Source: CAD feature listing. Evaluate the final solid. Frame: model axes, mm. Give positions to 0.01 mm unless a question says otherwise; leave off trailing zeros. Write each loop counter-clockwise with the first axis right and the second up, starting at its lowest first coordinate (ties: lowest second). Pieces come first, ordered by that corner, then holes. Notation, with made-up numbers: (83, -27.75) -> (110, -27.75) arc R27 ccw to (110, -11.75) -> close; hole circle Ø8 at (29.5, 15). An arc over 180 degrees is marked (long way). Answer as a JSON object with one key per item and string values. Group by question number.
Item 1: Section query B-B on x = 0. Return the cut outline in (y, z), plus the area to 3 significant figures.
Item 2: Section query A-A on y = 0. Return the cut outline in (x, z).
Item 3: First-contact query: pin 1 Ø3.5 at (x, y) = (-26.63, -8.65) entering from +Z; pin 2 Ø1.5 at (x, y) = (2, 15.5) entering from -Z; pin 3 Ø1 at (y, z) = (-8.5, 1) entering from -X; pin 4 Ø1 at (y, z) = (-23, 0.5) entering from -X. Flat tips, straight axial feed; report the tip coordinate or a pass-through.
Item 4: Pull-direction query (Y, two-part tool) for faces 1 (the face through (-2.93, -13.18, 1.97)), 2 (the face through (14, 0, 4)), 3 (the face through (31, 9.76, 1.97)); classes: pulls with the +Y half, pulls with the -Y half, needs draft (parallel to the pull), parting line crosses it, or undercut.
Item 5: Section query C-C on z = 3.1. Return the cut outline in (x, y), plus the area to 3 significant figures.
Item 6: Ray query, probe 1 along Y at (x, z) = (0, 2.2); probe 2 along X at (y, z) = (21.5, 0.8); probe 3 along X at (y, z) = (7.5, 3.15). Return the intervals inside material, ascending. Write a range as from..to.
Item 7: Section query D-D on x = 11.5. Return the cut outline in (y, z).
from build123d import *

# Parameters (mm, degrees)
SKETCH_1_R      = 32.5
SKETCH_1_R_2    = 13.5
SKETCH_1_R_3    = 2
EXTRUDE_1_DEPTH = 4


with BuildPart() as part:
    # 草图1 → 凸台-拉伸1 (new body)
    with BuildSketch(Plane.XY):
        Circle(SKETCH_1_R)
        Circle(SKETCH_1_R_2, mode=Mode.SUBTRACT)
        with Locations((0, -28)):
            Circle(SKETCH_1_R_3, mode=Mode.SUBTRACT)
        with Locations((-26.629582456, -8.652475842)):
            Circle(SKETCH_1_R_3, mode=Mode.SUBTRACT)
        with Locations((-16.457987064, 22.652475842)):
            Circle(SKETCH_1_R_3, mode=Mode.SUBTRACT)
        with Locations((16.457987064, 22.652475842)):
            Circle(SKETCH_1_R_3, mode=Mode.SUBTRACT)
        with Locations((26.629582456, -8.652475842)):
            Circle(SKETCH_1_R_3, mode=Mode.SUBTRACT)
    extrude(amount=EXTRUDE_1_DEPTH)


solid = part.part
Worked answers:
{
 "1": {"outline": "(-32.5, 0) -> (-30, 0) -> (-30, 4) -> (-32.5, 4) -> close; (-26, 0) -> (-13.5, 0) -> (-13.5, 4) -> (-26, 4) -> close; (13.5, 0) -> (32.5, 0) -> (32.5, 4) -> (13.5, 4) -> close", "area": "136 mm^2"},
 "2": {"outline": "(-32.5, 0) -> (-13.5, 0) -> (-13.5, 4) -> (-32.5, 4) -> close; (13.5, 0) -> (32.5, 0) -> (32.5, 4) -> (13.5, 4) -> close"},
 "3": {"pin 1": "through", "pin 2": "z = 0", "pin 3": "x = -31.5", "pin 4": "x = -23.45"},
 "4": {"face 1": "undercut", "face 2": "needs draft", "face 3": "parting line crosses it"},
 "5": {"outline": "circle Ø65 at (0, 0); hole circle Ø4 at (-26.63, -8.65); hole circle Ø4 at (-16.46, 22.65); hole circle Ø27 at (0, 0); hole circle Ø4 at (0, -28); hole circle Ø4 at (16.46, 22.65); hole circle Ø4 at (26.63, -8.65)", "area": "2,680 mm^2"},
 "6": {"probe 1": "-32.5..-30, -26..-13.5, 13.5..32.5", "probe 2": "-24.37..-18.09, -14.82..14.82, 18.09..24.37", "probe 3": "-31.62..-11.22, 11.22..31.62"},
 "7": {"outline": "(-30.4, 0) -> (-7.07, 0) -> (-7.07, 4) -> (-30.4, 4) -> close; (7.07, 0) -> (30.4, 0) -> (30.4, 4) -> (7.07, 4) -> close"}
}
